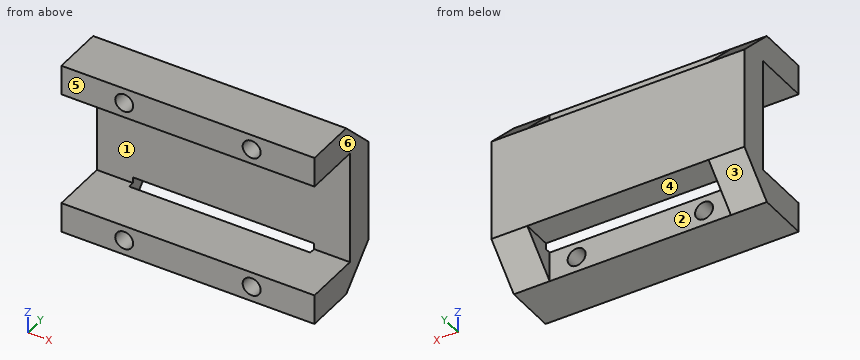
from build123d import *

# Parameters (mm, degrees)
F1_DEPTH = 42.3
F2_W     = 30.3
F2_H     = 6
F3_DEPTH = 6
F4_SIZE  = 6
F5_R     = 1.5
F6_DEPTH = 8.501
F7_R     = 1.5
F8_DEPTH = 8.501


# Not quite as in the source:
# - a feature names something its author has since deleted; it is built from what else it names


with BuildPart() as f1:
    # F0 (on Right) → F1 (new body)
    with BuildSketch(Plane.YZ):
        Polygon((0, 9.5), (9.5, 9.5), (9.5, -9.5), (0, -9.5), (0, -14.5), (14.5, -14.5), (14.5, 14.5), (0, 14.5), align=None)
    extrude(amount=F1_DEPTH)

    # F2 (on face) → F3 (cut)
    with BuildSketch(Plane(origin=(0, 14.5, 0), x_dir=(-1, 0, 0), z_dir=(0, 1, 0))):
        with Locations((-21.15, 11.5)):
            Rectangle(F2_W, F2_H)
        with Locations((-21.15, -11.5)):
            Rectangle(F2_W, F2_H)
    extrude(amount=-F3_DEPTH, mode=Mode.SUBTRACT)

    # F4
    f4_edges = [f1.edges().sort_by_distance(p)[0] for p in [
        (3, 14.5, -14.5),
        (39.3, 14.5, -14.5),
        (39.3, 14.5, 14.5),
        (3, 14.5, 14.5),
    ]]
    chamfer(f4_edges, length=F4_SIZE)

    # F5 (on face) → F6 (cut, through all)
    with BuildSketch(Plane(origin=(0, 8.5, 0), x_dir=(-1, 0, 0), z_dir=(0, 1, 0))):
        with Locations((-31.8, 12)):
            Circle(F5_R)
        with Locations((-10.5, 12)):
            Circle(F5_R)
    extrude(amount=-F6_DEPTH, mode=Mode.SUBTRACT)

    # F7 (on face) → F8 (cut, through all)
    with BuildSketch(Plane(origin=(0, 8.5, 0), x_dir=(-1, 0, 0), z_dir=(0, 1, 0))):
        with Locations((-31.8, -12)):
            Circle(F7_R)
        with Locations((-10.5, -12)):
            Circle(F7_R)
    extrude(amount=-F8_DEPTH, mode=Mode.SUBTRACT)


solid = f1.part
Verification items for the finished model (mm, model axes). Face numbers are marked on the shaded views. A direction names the side the tool comes from. Coordinates: 2 decimals unless noted, no trailing zeros. Order: outer loops, then holes, each group sorted by start corner. A loop starts at its lowest first (then second) coordinate and runs counter-clockwise, first axis right, second up. Notation, with made-up numbers: M 18,80.5 L 53,80.5 A14 ccw 53,101.5 Z; hole C -32.5,30 d1. An arc over 180 degrees is marked long. Write each question's results on one line, items separated by ' | '.
1) Scan lines: line 1 along Z through (x, y) = (10.5, 6.5); line 2 along Z through (x, y) = (16, 8); line 3 along Z through (x, y) = (11, 1.25). Record each from-to range of solid material in increasing order. Write a range as [from, to].
Solved:
line 1: z = [-14.5, -13.5], [-10.5, -9.5], [9.5, 10.5], [13.5, 14.5] | line 2: z = [-14.5, -9.5], [9.5, 14.5] | line 3: z = [-14.5, -13.41], [-10.59, -9.5], [9.5, 10.59], [13.41, 14.5]
2) Release check for a two-part mould opening along X. For the marked faces 4, 5 and 6 record: pulls with the +X half, pulls with the -X half, needs draft (parallel to the pull), parting line crosses it, or undercut.
Solved:
face 4: undercut | face 5: needs draft | face 6: pulls with the +X half
3) Access from +Z, -Z, +X, -X, +Y, -Y to the whole of each face (thin tool, end or side, straight path). Record for the marked faces 1, 2 and 3.
Solved:
face 1: +X, -X, -Y | face 2: +Z, -Z, +Y | face 3: -Z, +X, -X, +Y
4) Gauge pin test, flat ends, axial feed: pin 1 Ø5 at (y, z) = (12.5, -10.5) entering from -X; pin 2 Ø4 at (x, z) = (10.5, 12) entering from +Y; pin 3 Ø5.5 at (x, z) = (17, -3.5) entering from -Y; pin 4 Ø2.5 at (x, y) = (28.5, 12.5) entering from -Z. Record the tip position at first contact, or that the pin passes through.
Solved:
pin 1: stops at x = 0 | pin 2: stops at y = 8.5 | pin 3: stops at y = 9.5 | pin 4: stops at z = -8.5
5) Section check A-A on y = 4.25. Record the cut outline in (x, z), plus the area to 3 significant figures.
Solved:
outline: M 0,-14.5 L 42.3,-14.5 L 42.3,-9.5 L 0,-9.5 Z; M 0,9.5 L 42.3,9.5 L 42.3,14.5 L 0,14.5 Z; hole C 10.5,-12 d3; hole C 10.5,12 d3; hole C 31.8,-12 d3; hole C 31.8,12 d3 | area: 395 mm²
6) Section check B-B on x = 10.5. Record the cut outline in (y, z), plus the area to 3 significant figures.
Solved:
outline: M 0,-14.5 L 8.5,-14.5 L 8.5,-13.5 L 0,-13.5 Z; M 0,-10.5 L 8.5,-10.5 L 8.5,-9.5 L 0,-9.5 Z; M 0,9.5 L 8.5,9.5 L 8.5,10.5 L 0,10.5 Z; M 0,13.5 L 8.5,13.5 L 8.5,14.5 L 0,14.5 Z; M 9.5,-8.5 L 14.5,-8.5 L 14.5,8.5 L 9.5,8.5 Z | area: 119 mm²
7) Section check C-C on x = 35. Record the cut outline in (y, z), plus the area to 3 significant figures.
Solved:
outline: M 0,-14.5 L 8.5,-14.5 L 8.5,-9.5 L 0,-9.5 Z; M 0,9.5 L 8.5,9.5 L 8.5,14.5 L 0,14.5 Z; M 9.5,-8.5 L 14.5,-8.5 L 14.5,8.5 L 9.5,8.5 Z | area: 170 mm²
8) Section check D-D on z = 12. Record the cut outline in (x, y).
Solved:
outline: M 0,0 L 9,0 L 9,8.5 L 6,8.5 L 6,11 L 0,11 Z; M 12,0 L 30.3,0 L 30.3,8.5 L 12,8.5 Z; M 33.3,0 L 42.3,0 L 42.3,11 L 36.3,11 L 36.3,8.5 L 33.3,8.5 Z
